The model under review builds one solid part; all positions refer to its coordinate system, in mm. A direction names the side the tool comes from. Give positions to 0.01 mm unless a question says otherwise; leave off trailing zeros. Order: outer loops, then holes, each group sorted by start corner. A loop starts at its lowest first (then second) coordinate and runs counter-clockwise, first axis right, second up. Notation, with made-up numbers: (-14, -26.5) - (0, -26.5) arc R22 cw to (0, -5.5) - close; hole circle Ø10 at (-33, 20.25). An arc over 180 degrees is marked (long way). Use CSV: the item, a comma, the result in double quotes.
Autodesk Inventor part; units mm, degrees
ref_plane "YZ Plane" through (0, 0, 0) normal (1, 0, 0) x (0, 1, 0)
ref_plane "XZ Plane" through (0, 0, 0) normal (0, 1, 0) x (-1, 0, 0)
ref_plane "XY Plane" through (0, 0, 0) normal (0, 0, 1) x (1, 0, 0)
sketch "Sketch1" plane through (0, 0, 0) normal (0, 1, 0) x (-1, 0, 0)
  line L0 (0, 0) -> (406.4, 0)
  line L1 (406.4, 0) -> (406.4, -469.9)
  line L2 (406.4, -469.9) -> (0, -469.9)
  line L3 (0, -469.9) -> (0, 0)
  dimension "d0" = 406.4
  dimension "d1" = 469.9
extrude "Extrusion1" add sketch "Sketch1" along normal blind 1.905
sketch "Sketch2" plane through (0, 1.905, 0) normal (0, 1, 0) x (1, 0, 0)
  line L0 (-406.4, 469.9) -> (-406.4, 0)
  line L1 (0, 0) -> (0, 469.9)
  line L2 (-406.4, 0) -> (0, 0)
  line L3 (0, 0) -> (0, 1.905)
  line L4 (-1.905, 1.905) -> (-406.4, 1.905)
  line L5 (-406.4, 1.905) -> (-406.4, 0)
  line L6 (0, 469.9) -> (-406.4, 469.9)
  line L7 (0, 0) -> (-52.705, 0)
  line L8 (-1.905, 1.905) -> (-1.905, 467.995)
  line L9 (-1.905, 469.9) -> (0, 469.9)
  line L10 (0, 469.9) -> (0, 0)
  line L11 (0, 469.9) -> (-406.4, 469.9)
  line L12 (-406.4, 469.9) -> (-406.4, 467.995)
  line L13 (-406.4, 467.995) -> (-1.905, 467.995)
  line L14 (0, 467.995) -> (0, 469.9)
  dimension "d4" = 1.905
  dimension "d5" = 1.905
  dimension "d6" = 1.905
  dimension "d13" = 1.905
extrude "Extrusion2" add sketch "Sketch2" along normal blind 177.8 contours L6 L1 L2 L0 L4 L8 L13
sketch "Sketch3" plane through (0, 179.705, 0) normal (0, 1, 0) x (1, 0, 0)
  line L0 (-1.905, 467.995) -> (-1.905, 1.905)
  line L1 (0, 469.9) -> (0, 0)
  line L2 (-1.905, 342.9) -> (0, 342.9)
  line L3 (0, 342.9) -> (0, 127)
  line L4 (0, 127) -> (-1.905, 127)
  line L5 (-1.905, 127) -> (-1.905, 342.9)
  line L6 (-406.4, 0) -> (0, 0)
  line L7 (0, 469.9) -> (-406.4, 469.9)
  dimension "d9" = 127
  dimension "d10" = 127
extrude "Extrusion3" cut sketch "Sketch3" against normal blind 177.8
properties part number "hopper_bottom2"
Item 1: Take a section at D-D, the plane z = -306. Give the boundary of the cut face in (x, y) (3 decimals).
Results list:
outline,"(-406.4, 0) - (0, 0) - (0, 1.905) - (-406.4, 1.905) - close"
Item 2: Mouldability with a two-part tool opening along Z and no side actions: class faces 1 (the face through (-1.905, 90, -64)), 2 (the face through (-207, 90, -467.995)), 3 (the face through (-206, 89, -469.9)), 4 (the face through (-200, 0, -232)) as pulls with the +Z half, pulls with the -Z half, needs draft (parallel to the pull), parting line crosses it, or undercut.
Results list:
face 1,"undercut"
face 2,"undercut"
face 3,"pulls with the -Z half"
face 4,"needs draft"
Item 3: Clearance check with flat-ended pins moving along their axes: pin 1 (6 mm diameter, centred on x = -314, y = 100, fed in from +Z); pin 2 (8 mm diameter, centred on x = -115.5, z = -89, fed in from +Y) (3 decimals). State where each tip first meets the part, or that it passes through.
Results list:
pin 1,"stops at z = 0"
pin 2,"stops at y = 1.905"
Item 4: Take a section at B-B, the plane x = -165. Give the boundary of the cut face in (y, z) (3 decimals).
Results list:
outline,"(0, -469.9) - (179.705, -469.9) - (179.705, -467.995) - (1.905, -467.995) - (1.905, -1.905) - (179.705, -1.905) - (179.705, 0) - (0, 0) - close"
Item 5: Tool access review of faces 5 (the face through (-201, 90, -1.905)), 6 (the face through (0, 89, -395)): name each direction out of +Z, -Z, +X, -X, +Y, -Y from which nothing blocks a thin tool from reaching the whole face with its end or side.
Results list:
face 5,"-X, +Y"
face 6,"+Z, -Z, +X, +Y, -Y"
Item 6: Take a section at A-A, the plane y = 122.5. Give the boundary of the cut face in (x, z) (3 decimals), and give its area (4 significant figures).
Results list:
outline,"(-406.4, -469.9) - (0, -469.9) - (0, -342.9) - (-1.905, -342.9) - (-1.905, -467.995) - (-406.4, -467.995) - close; (-406.4, -1.905) - (-1.905, -1.905) - (-1.905, -127) - (0, -127) - (0, 0) - (-406.4, 0) - close"
area,"2,025 mm2"
Item 7: Wall thickness on L1, parallel to Z at x = -34.5, y = 151 (3 decimals); L2, parallel to Y at x = -332.5, z = -89 (3 decimals); L3, parallel to X at y = 37, z = -116 (3 decimals): over which ranges is each line inside the solid? List them lowest first.
Results list:
L1,"z = -469.9 to -467.995, -1.905 to 0"
L2,"y = 0 to 1.905"
L3,"x = -1.905 to 0"
Item 8: Take a section at C-C, the plane z = -55. Give the boundary of the cut face in (x, y) (3 decimals), and give its area (3 significant figures).
Results list:
outline,"(-406.4, 0) - (0, 0) - (0, 179.705) - (-1.905, 179.705) - (-1.905, 1.905) - (-406.4, 1.905) - close"
area,"1,110 mm2"
